from build123d import *

# Parameters (mm, degrees)
AUFSATZ_LINEAR_AUSTRAGEN1_DEPTH = 5
AUFSATZ_LINEAR_AUSTRAGEN2_DEPTH = 5
SCHNITT_LINEAR_AUSTRAGEN1_DEPTH = 384.76425055
SCHNITT_LINEAR_AUSTRAGEN2_DEPTH = 384.76425055
SKIZZE5_R                       = 1.6
SCHNITT_LINEAR_AUSTRAGEN3_DEPTH = 384.666521865
FASE1_SIZE                      = 2
AUFSATZ_LINEAR_AUSTRAGEN3_DEPTH = 21.5
SKIZZE7_R                       = 2.1
SCHNITT_LINEAR_AUSTRAGEN4_DEPTH = 385.548111424
AUFSATZ_LINEAR_AUSTRAGEN4_DEPTH = 24.2
FASE2_SIZE                      = 2.5


with BuildPart() as part:
    # Skizze1 → Aufsatz-Linear austragen1 (new body)
    with BuildSketch(Plane(origin=(0, 0, 0), x_dir=(1, 0, 0), z_dir=(0, 1, 0))):
        with BuildLine():
            Line((0, 0), (290, 0))
            ThreePointArc((290, 0), (251.147367097, 145), (145, 251.147367097))
            Line((145, 251.147367097), (0, 0))
        make_face()
    extrude(amount=AUFSATZ_LINEAR_AUSTRAGEN1_DEPTH)

    # Skizze2 → Aufsatz-Linear austragen2 (add)
    with BuildSketch(Plane(origin=(0, 5, 0), x_dir=(1, 0, 0), z_dir=(0, 1, 0))):
        with BuildLine():
            Line((0, 0), (149.9, 0))
            ThreePointArc((149.9, 0), (129.817208027, 74.95), (74.95, 129.817208027))
            Line((74.95, 129.817208027), (0, 0))
        make_face()
    extrude(amount=AUFSATZ_LINEAR_AUSTRAGEN2_DEPTH)

    # Skizze3 → Schnitt-Linear austragen1 (cut, through all)
    with BuildSketch(Plane(origin=(0, 10, 0), x_dir=(1, 0, 0), z_dir=(0, 1, 0))):
        Polygon((26.2, 45.379731158), (94.633560231, 84.889865579), (120.833560231, 39.510134421), (52.4, 0), (0, 0), align=None)
    extrude(amount=-SCHNITT_LINEAR_AUSTRAGEN1_DEPTH, mode=Mode.SUBTRACT)

    # Skizze4 → Schnitt-Linear austragen2 (cut, through all)
    with BuildSketch(Plane(origin=(0, 10, 0), x_dir=(1, 0, 0), z_dir=(0, 1, 0))):
        with BuildLine():
            Line((100, 0), (0, 0))
            Line((0, 0), (50, 86.602540378))
            ThreePointArc((50, 86.602540378), (86.602540378, 50), (100, 0))
        make_face()
    extrude(amount=-SCHNITT_LINEAR_AUSTRAGEN2_DEPTH, mode=Mode.SUBTRACT)

    # Skizze5 → Schnitt-Linear austragen3 (cut, through all)
    with BuildSketch(Plane(origin=(0, 5, 0), x_dir=(1, 0, 0), z_dir=(0, 1, 0))):
        with Locations(Location((95.879925069, 124.953151096, 0), (0, 0, 270))):
            Circle(SKIZZE5_R)
        with Locations(Location((224.122318632, 171.975103695, 0), (0, 0, 270))):
            Circle(SKIZZE5_R)
        with Locations(Location((145.511026371, 60.272640598, 0), (0, 0, 270))):
            Circle(SKIZZE5_R)
        with Locations(Location((280.083173338, 36.873649302, 0), (0, 0, 270))):
            Circle(SKIZZE5_R)
    extrude(amount=-SCHNITT_LINEAR_AUSTRAGEN3_DEPTH, mode=Mode.SUBTRACT)

    # Fase1
    fase1_edges = [part.edges().sort_by_distance(p)[0] for p in [
        (95.879925069, 0, -126.553151096),
        (224.122318632, 0, -173.575103695),
        (145.511026371, 0, -61.872640598),
        (280.083173338, 0, -38.473649302),
    ]]
    chamfer(fase1_edges, length=FASE1_SIZE)

    # Skizze6 → Aufsatz-Linear austragen3 (add)
    with BuildSketch(Plane(origin=(0, 5, 0), x_dir=(1, 0, 0), z_dir=(0, 1, 0))):
        Polygon((207.976550727, 76.774047358), (219.234880976, 83.274047358), (209.234880976, 100.594555434), (197.976550727, 94.094555434), align=None)
    extrude(amount=AUFSATZ_LINEAR_AUSTRAGEN3_DEPTH)

    # Skizze7 → Schnitt-Linear austragen4 (cut, through all)
    with BuildSketch(Plane(origin=(0, 26.5, 0), x_dir=(1, 0, 0), z_dir=(0, 1, 0))):
        with Locations(Location((206.105715851, 93.014428415, 0), (0, 0, 270))):
            Circle(SKIZZE7_R)
        with Locations(Location((211.105715851, 84.354174377, 0), (0, 0, 270))):
            Circle(SKIZZE7_R)
    extrude(amount=-SCHNITT_LINEAR_AUSTRAGEN4_DEPTH, mode=Mode.SUBTRACT)

    # Skizze9 → Aufsatz-Linear austragen4 (add)
    with BuildSketch(Plane(origin=(0, 5, 0), x_dir=(1, 0, 0), z_dir=(0, 1, 0))):
        Polygon((197.976550727, 94.094555434), (207.976550727, 76.774047358), (206.244499919, 75.774047358), (196.244499919, 93.094555434), align=None)
        Polygon((219.234880976, 83.274047358), (220.966931784, 84.274047358), (210.966931784, 101.594555434), (209.234880976, 100.594555434), align=None)
    extrude(amount=AUFSATZ_LINEAR_AUSTRAGEN4_DEPTH)

    # Fase2
    fase2_edges = [part.edges().sort_by_distance(p)[0] for p in [
        (206.105715851, 0, -95.114428415),
        (211.105715851, 0, -86.454174377),
    ]]
    chamfer(fase2_edges, length=FASE2_SIZE)


solid = part.part
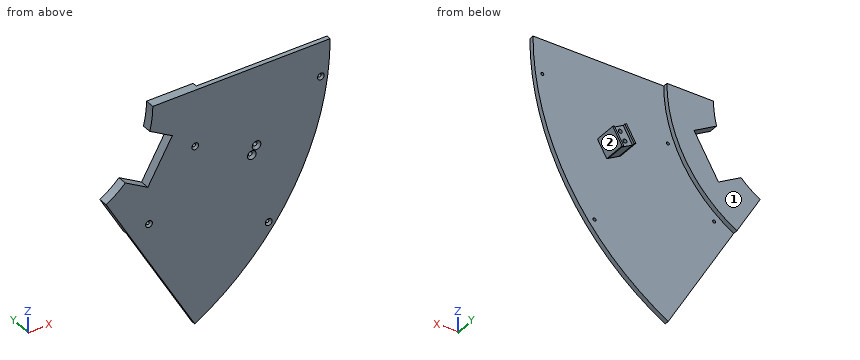
Model file for the job. Use its own axes, mm. Face numbers are marked on the shaded views. Give positions to 0.01 mm unless a question says otherwise; leave off trailing zeros. Order: outer loops, then holes, each group sorted by start corner. A loop starts at its lowest first (then second) coordinate and runs counter-clockwise, first axis right, second up. Notation, with made-up numbers: (-33, -31) - (11, -31) arc R25 cw to (11, 7) - close; hole circle Ø8 at (56.5, 11.5). An arc over 180 degrees is marked (long way). Return JSON: item names as keys, results as strings.
1) Flat gauge pins, fed straight in: P1, Ø12, axis at x = 185, z = -48.5, coming from the +Y side; P2, Ø6, axis at x = 208, y = 4, coming from the -Z side; P3, Ø8, axis at y = 12.5, z = -52.5, coming from the +X side. Where does each tip first touch, or does it go through?
Geometry says:
{"P1": "y = 5", "P2": "z = -205.12", "P3": "x = 141.53"}
2) Cut at B-B, the plane x = 89. Give the cut face in (y, z), plus the area to 3 significant figures.
Geometry says:
{"outline": "(0, -154.15) - (5, -154.15) - (5, -120.62) - (10, -120.62) - (10, -81.64) - (0, -81.64) - close", "area": "557 mm²"}
3) Pull direction Z, two halves, no side cores. Call the marked faces 1 and 2: pulls with the +Z half, pulls with the -Z half, needs draft (parallel to the pull), parting line crosses it, or undercut.
Geometry says:
{"face 1": "needs draft", "face 2": "pulls with the -Z half"}
4) Cut at A-A, the plane y = 22.25. Give the cut face in (x, z).
Geometry says:
{"outline": "(196.24, -93.09) - (210.97, -101.59) - (220.97, -84.27) - (206.24, -75.77) - close; hole circle Ø4.2 at (206.11, -93.01); hole circle Ø4.2 at (211.11, -84.35)"}
5) Cut at D-D, the plane x = 161. Give the cut face in (y, z).
Geometry says:
{"outline": "(0, -241.2) - (5, -241.2) - (5, 0) - (0, 0) - close"}
6) Probe line 1 (Y direction, x = 153, z = -142); line 2 (Y direction, x = 126, z = -25.5); line 3 (X direction, y = 10.25, z = -89.5). List the from-to ranges inside material, lowest first. Write a range as from..to.
Geometry says:
{"line 1": "0..5", "line 2": "0..10", "line 3": "198.32..217.95"}
7) Cut at C-C, the plane z = -114. Give the cut face in (x, y).
Geometry says:
{"outline": "(65.82, 0) - (266.65, 0) - (266.65, 5) - (97.33, 5) - (97.33, 10) - (65.82, 10) - close"}
